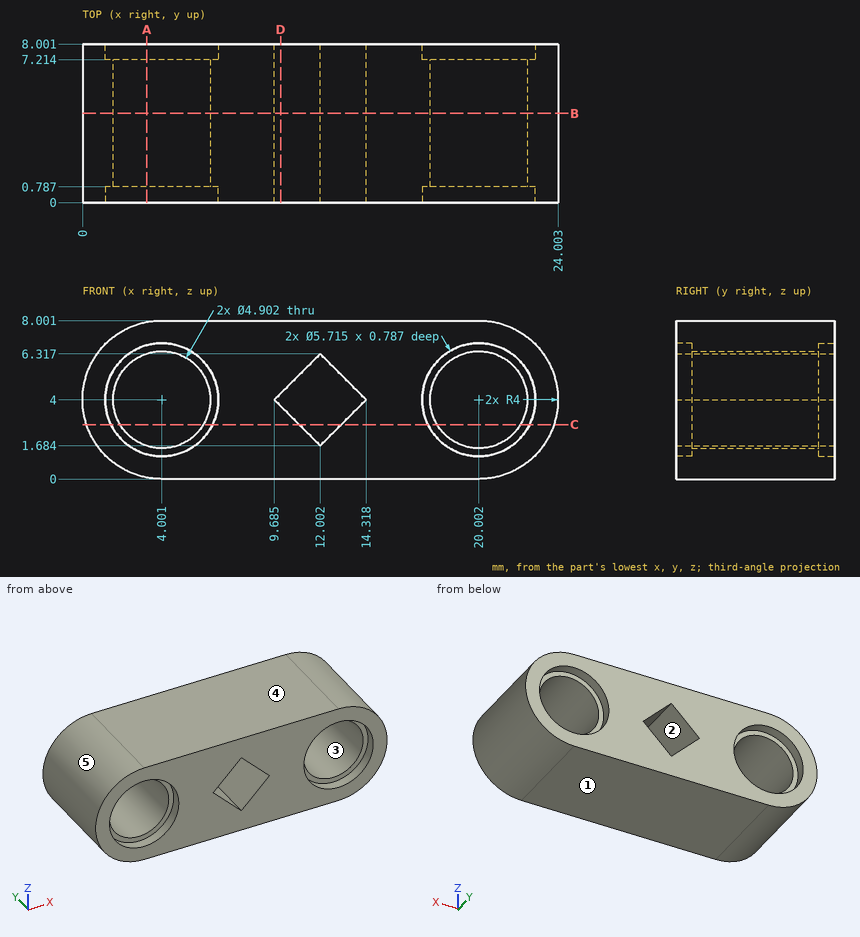
Could you check a few things on this drawing? It's one solid part, dimensions in mm from its lowest x, y, z. A direction names the side the tool comes from. Coordinates: 2 decimals unless noted, no trailing zeros. Write each loop counter-clockwise with the first axis right and the second up, starting at its lowest first coordinate (ties: lowest second). Pieces come first, ordered by that corner, then holes. Notation, with made-up numbers: (44, 50.5) - (84, 50.5) arc R17 cw to (84, 59.5) - close; hole circle Ø1 at (24.5, 88.25). An arc over 180 degrees is marked (long way). Put each result on its own line as item: value. Start each with the question number.
Q1. Please list where these lines run through material, in increasing order: L1, parallel to X at y = 7, z = 3.25 (1 decimal); L2, parallel to X at y = 4, z = 4.5 (1 decimal); L3, parallel to Z at x = 3.75, y = 3.75.
Q2. Thinking about a two-plate mould opening in X: for the marked faces 3, 4 and 5, which applies, pulls with the +X half, pulls with the -X half, needs draft (parallel to the pull), parting line crosses it, or undercut?
Q3. Which directions (+Z, -Z, +X, -X, +Y, -Y) give clear straight access to the entire face, cutting with the end or side of a thin tool? Please do the marked faces 1 and 2.
Q4. I want a section at A-A on x = 3.25. Write out the boundary of the cut face in (y, z), plus the area to 3 significant figures.
Q5. I'm going to push flat-ended pins straight in: P1, Ø1.7, axis at x = 18.5, z = 2.5, coming from the +Y side; P2, Ø3, axis at x = 3, z = 4, coming from the +Y side; P3, Ø1.5, axis at y = 6, z = 2, coming from the +X side. Where does each tip first touch, or does it pass through?
Q6. I want a section at B-B on y = 4.5. Write out the boundary of the cut face in (x, z) (1 decimal).
Q7. I want a section at D-D on x = 10. Write out the boundary of the cut face in (y, z) (1 decimal).
Q8. I want a section at C-C on z = 2.75. Count the separate pieces of the cut face and the enclosed holes in it, plus the area to 3 significant figures.
Checks:
1. L1: 0.1 to 1.7, 6.3 to 10.4, 13.6 to 17.7, 22.3 to 23.9
1. L2: 0 to 1.6, 6.4 to 10.2, 13.8 to 17.6, 22.4 to 24
1. L3: 0.01 to 1.56, 6.44 to 7.99
2. face 3: undercut
2. face 4: needs draft
2. face 5: pulls with the -X half
3. face 1: -Z, +X, -X, +Y, -Y
3. face 2: +Y, -Y
4. outline: (0, 0.07) - (8, 0.07) - (8, 1.24) - (7.21, 1.24) - (7.21, 1.67) - (0.79, 1.67) - (0.79, 1.24) - (0, 1.24) - close; (0, 6.76) - (0.79, 6.76) - (0.79, 6.33) - (7.21, 6.33) - (7.21, 6.76) - (8, 6.76) - (8, 7.93) - (0, 7.93) - close
4. area: 24.2 mm²
5. P1: y = 8
5. P2: y = 7.21
5. P3: x = 23.8
6. outline: (4, 0) - (20, 0) arc R4 ccw to (20, 8) - (4, 8) arc R4 ccw to start; hole circle Ø4.9 at (4, 4); hole (9.7, 4) - (12, 1.7) - (14.3, 4) - (12, 6.3) - close; hole circle Ø4.9 at (20, 4)
7. outline: (0, 0) - (8, 0) - (8, 3.7) - (0, 3.7) - close; (0, 4.3) - (8, 4.3) - (8, 8) - (0, 8) - close
8. separate pieces: 4
8. enclosed holes: 0
8. area: 101 mm²
